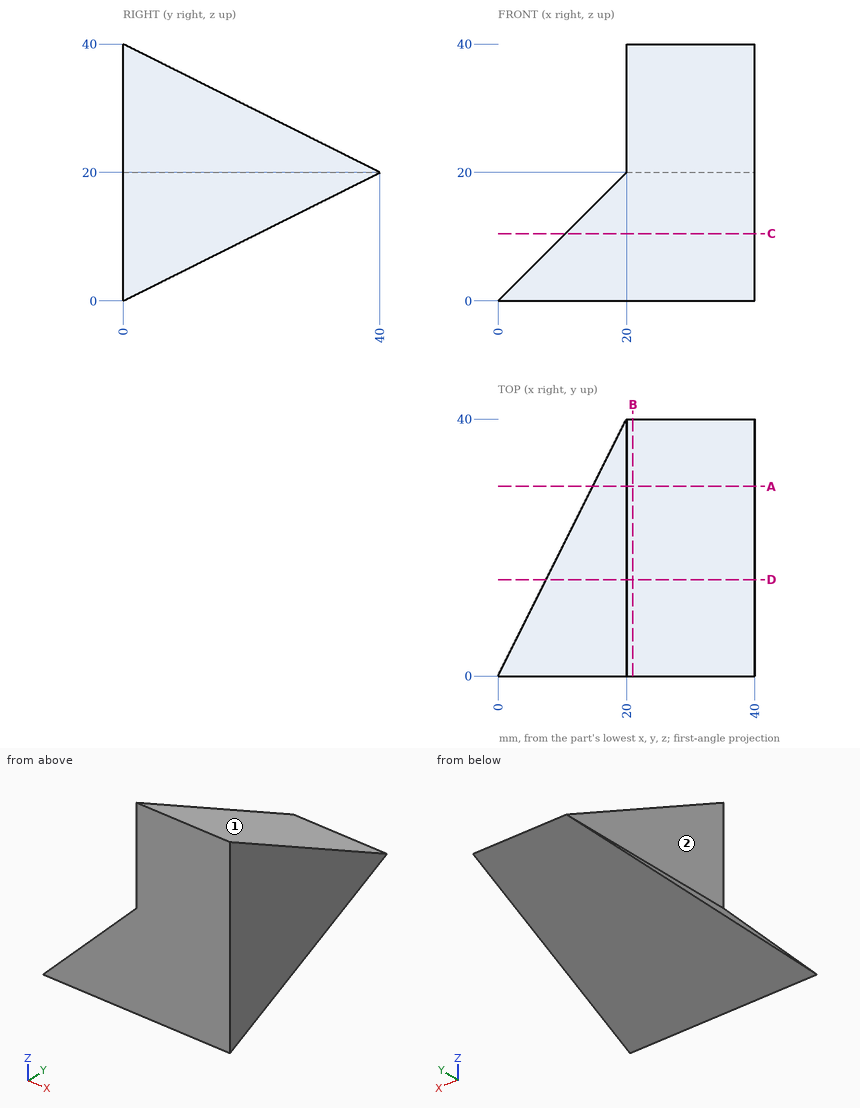
Print and shaded views of the part. All mm, measured from the part's lowest x, y and z. A direction names the side the tool comes from. Round coordinates to 2 decimals unless told otherwise and drop trailing zeros. Write each loop counter-clockwise with the first axis right and the second up, starting at its lowest first coordinate (ties: lowest second). Pieces come first, ordered by that corner, then holes.
Item 1: Drop flat-ended pins along their axis: pin 1 Ø8 at (x, y) = (20.5, 35.5) entering from +Z; pin 2 Ø10 at (x, y) = (23.5, 19) entering from -Z; pin 3 Ø5 at (x, y) = (31, 24.5) entering from -Z. Give the stop position or say it passes through.
Results:
pin 1: stops at z = 24.25
pin 2: stops at z = 7
pin 3: stops at z = 11
Item 2: Cut at C-C, the plane z = 10.5. Give the cut face in (x, y), plus the area to 4 significant figures.
Results:
outline: (10.5, 0) - (40, 0) - (40, 21) - (10.5, 21) - close
area: 619.5 mm2
Item 3: Cut at B-B, the plane x = 21. Give the cut face in (y, z), plus the area to 3 significant figures.
Results:
outline: (0, 0) - (40, 20) - (0, 40) - close
area: 800 mm2
Item 4: Probe L1, parallel to X at y = 10.5, z = 22; L2, parallel to X at y = 16.5, z = 12; L3, parallel to Y at x = 34, z = 37. List the from-to ranges inside material, lowest first.
Results:
L1: x = 20 to 40
L2: x = 12 to 40
L3: y = 0 to 6
Item 5: Cut at A-A, the plane y = 29.5. Give the cut face in (x, z), plus the area to 3 significant figures.
Results:
outline: (14.75, 14.75) - (40, 14.75) - (40, 25.25) - (20, 25.25) - (20, 20) - close
area: 224 mm2
Item 6: Which spindle directions (+Z, -Z, +X, -X, +Y, -Y) get a long thin tool onto all of the face, cutting with end or side? Do the marked faces 1 and 2. Say none if no direction does.
Results:
face 1: +Z, +X, -X, +Y
face 2: +Z, -X, +Y, -Y
Item 7: Cut at D-D, the plane y = 15. Give the cut face in (x, z), plus the area to 3 significant figures.
Results:
outline: (7.5, 7.5) - (40, 7.5) - (40, 32.5) - (20, 32.5) - (20, 20) - close
area: 578 mm2
